Input: dimensioned drawing with shaded views. Units: mm. Origin: part minimum x, y, z. Give positions to 0.01 mm unless a question says otherwise; leave off trailing zeros. Write each loop counter-clockwise with the first axis right and the second up, starting at its lowest first coordinate (ties: lowest second). Pieces come first, ordered by that corner, then holes. Notation, with made-up numbers: M -28,7 L -12,7 A15 ccw -12,32 Z; hole C 31.25,24.25 d9. An arc over 180 degrees is marked long. Answer as a JSON object with one key per item and string values.
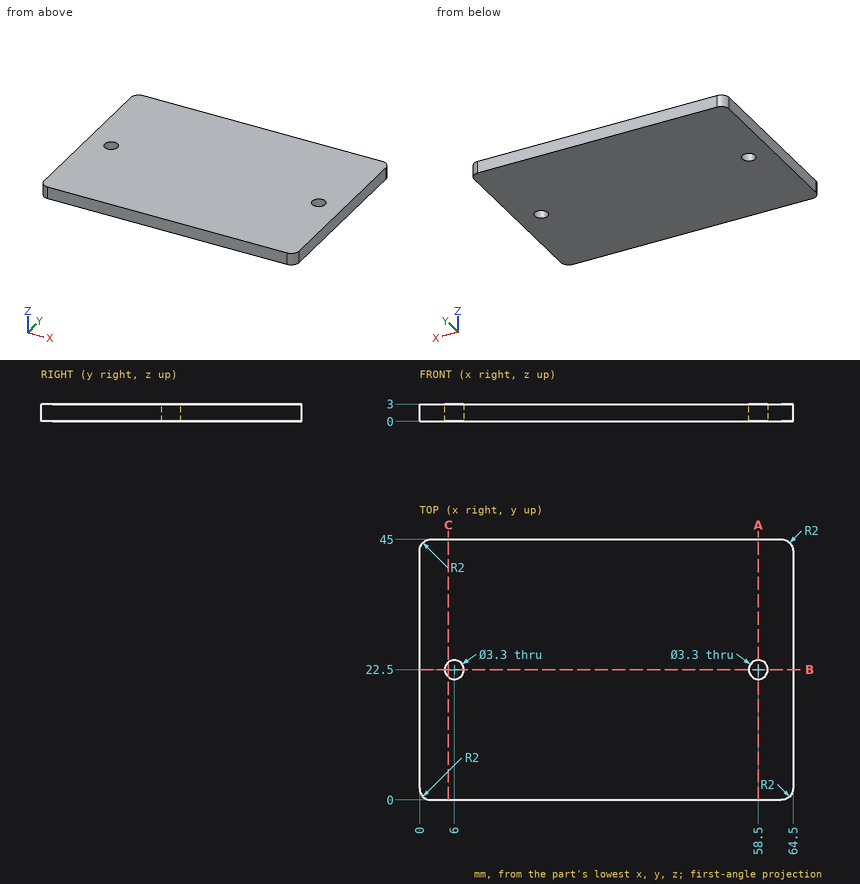
1) Line query: line 1 (Y direction, x = 58.5, z = 1.7). Output: solid intervals per line, ascending. Write a range as from..to.
Geometry check:
{"line 1": "y = 0..20.85, 24.15..45"}
2) Cut plane A-A on x = 58.5. Return loops of the section in (y, z), and give its area (3 significant figures).
Geometry check:
{"outline": "M 0,0 L 20.85,0 L 20.85,3 L 0,3 Z; M 24.15,0 L 45,0 L 45,3 L 24.15,3 Z", "area": "125 mm2"}
3) Cut plane B-B on y = 22.5. Return loops of the section in (x, z), and give its area (3 significant figures).
Geometry check:
{"outline": "M 0,0 L 4.35,0 L 4.35,3 L 0,3 Z; M 7.65,0 L 56.85,0 L 56.85,3 L 7.65,3 Z; M 60.15,0 L 64.5,0 L 64.5,3 L 60.15,3 Z", "area": "174 mm2"}
4) Cut plane C-C on x = 5. Return loops of the section in (y, z).
Geometry check:
{"outline": "M 0,0 L 21.19,0 L 21.19,3 L 0,3 Z; M 23.81,0 L 45,0 L 45,3 L 23.81,3 Z"}
